The model under review builds one solid part; all positions refer to its coordinate system, in mm. A direction names the side the tool comes from. Round coordinates to 2 decimals unless told otherwise and drop trailing zeros. Write each loop counter-clockwise with the first axis right and the second up, starting at its lowest first coordinate (ties: lowest second). Pieces come first, ordered by that corner, then holes.
Item 1: Add section A-A (x = -45.5). Give the boundary of the cut face in (y, z).
Item 2: Machinability: for faces 1 (the face through (-8.642, 13.555, -0.07)), 2 (the face through (24, -22, 0)), 3 (the face through (-36.3, -58, 2)), which of the approach directions +Z, -Z, +X, -X, +Y, -Y give a long, thin tool a straight path to every point of the face, cutting with its end or side? Answer none if there is none.
Item 3: Draft analysis for pull direction Y (two halves, no side actions). For faces 4 (the face through (-1, -73.8, 2)), 5 (the face through (0, 0, -5)), 6 (the face through (36.3, -59, 2)), state which applies: +Y half, -Y half, draft (parallel to the pull), parting line (faces both ways), or undercut.
Item 4: To check wall thickness, follow L1, parallel to Y at x = 0, z = 3.25 (3 decimals); L2, parallel to Z at x = -47, y = 2.5; L3, parallel to Y at x = -12, z = 1.5. State the ranges of each line that lie inside material, in increasing order.
Item 5: Clearance check with flat-ended pins moving along their axes: pin 1 Ø2.5 at (y, z) = (-54.5, 3) entering from -X; pin 2 Ø2 at (y, z) = (-35, -0.5) entering from +X; pin 3 Ø1.5 at (x, z) = (-38, 1.5) entering from +Y. State where each tip first meets the part, or that it passes through.
```python
from build123d import *

# Parameters (mm, degrees)
BOSS_EXTRUDE1_DEPTH = 5
SKETCH2_R           = 16.075
CUT_EXTRUDE1_DEPTH  = 33
BOSS_EXTRUDE2_START = 5
SKETCH3_R           = 21.075
SKETCH3_R_2         = 16.075
BOSS_EXTRUDE2_DEPTH = 5
BOSS_EXTRUDE3_START = 3
SKETCH4_R           = 21.075
BOSS_EXTRUDE3_DEPTH = 3
FILLET1_R           = 7
FILLET2_R           = 7


with BuildPart() as part:
    # Sketch1 → Boss-Extrude1 (new body)
    with BuildSketch(Plane.XY):
        with BuildLine():
            ThreePointArc((36.3, -43.034869583), (0, 56.3), (-36.3, -43.034869583))
            Line((-36.3, -43.034869583), (-36.3, -73.8))
            Line((-36.3, -73.8), (36.3, -73.8))
            Line((36.3, -73.8), (36.3, -43.034869583))
        make_face()
    extrude(amount=BOSS_EXTRUDE1_DEPTH)

    # Sketch2 → Cut-Extrude1 (cut)
    with BuildSketch(Plane(origin=(0, 0, 0), x_dir=(-1, 0, 0), z_dir=(0, 0, -1))):
        Circle(SKETCH2_R)
    extrude(amount=-CUT_EXTRUDE1_DEPTH, mode=Mode.SUBTRACT)

    # Sketch3 → Boss-Extrude2 (add)
    with BuildSketch(Plane(origin=(0, 0, 0), x_dir=(-1, 0, 0), z_dir=(0, 0, -1)).offset(BOSS_EXTRUDE2_START)):
        with Locations(Location((0, 0, 0), (0, 0, 180))):
            Circle(SKETCH3_R)
        Circle(SKETCH3_R_2, mode=Mode.SUBTRACT)
    extrude(amount=-BOSS_EXTRUDE2_DEPTH)

    # Sketch4 → Boss-Extrude3 (add)
    with BuildSketch(Plane(origin=(0, 0, -5), x_dir=(-1, 0, 0), z_dir=(0, 0, -1)).offset(BOSS_EXTRUDE3_START)):
        with Locations(Location((0, 0, 0), (0, 0, 180))):
            Circle(SKETCH4_R)
    extrude(amount=-BOSS_EXTRUDE3_DEPTH)

    # Fillet1
    fillet1_edges = [part.edges().sort_by_distance(p)[0] for p in [
        (-21.075, 0, 0),
    ]]
    fillet(fillet1_edges, radius=FILLET1_R)

    # Fillet2
    fillet2_edges = [part.edges().sort_by_distance(p)[0] for p in [
        (-21.075, 0, -8),
    ]]
    fillet(fillet2_edges, radius=FILLET2_R)


solid = part.part
```
Numbers:
1. outline: (-33.16, 0) - (33.16, 0) - (33.16, 5) - (-33.16, 5) - close
2. face 1: +Z
2. face 2: -Z
2. face 3: +Z, -Z, -X, -Y
3. face 4: -Y half
3. face 5: undercut
3. face 6: draft
4. L1: y = -73.8 to -16.075, 16.075 to 56.3
4. L2: z = 0 to 5
4. L3: y = -73.8 to -10.7, 10.7 to 55.01
5. pin 1: stops at x = -36.3
5. pin 2: stops at x = 44.77
5. pin 3: stops at y = 42.22
